from build123d import *

# Parameters (mm, degrees)
SKETCH2_R           = 12.954
BOSS_EXTRUDE1_DEPTH = 3.175
SKETCH3_R           = 5.969
BOSS_EXTRUDE2_DEPTH = 8.001
SKETCH4_R           = 2.794
SKETCH4_R_2         = 2.159
SKETCH4_R_3         = 1.397
BOSS_EXTRUDE3_DEPTH = 4.318


with BuildPart() as part:
    # Sketch2 → Boss-Extrude1 (new body)
    with BuildSketch(Plane(origin=(0, 0, 0), x_dir=(1, 0, 0), z_dir=(0, 1, 0))):
        with Locations(Location((0, 0, 0), (0, 0, 270))):
            Circle(SKETCH2_R)
    extrude(amount=BOSS_EXTRUDE1_DEPTH)

    # Sketch3 → Boss-Extrude2 (add)
    with BuildSketch(Plane(origin=(0, 3.175, 0), x_dir=(1, 0, 0), z_dir=(0, 1, 0))):
        with Locations(Location((0, 0, 0), (0, 0, 270))):
            Circle(SKETCH3_R)
    extrude(amount=BOSS_EXTRUDE2_DEPTH)

    # Sketch4 → Boss-Extrude3 (add)
    with BuildSketch(Plane(origin=(0, 11.176, 0), x_dir=(1, 0, 0), z_dir=(0, 1, 0))):
        with Locations(Location((0, 0, 0), (0, 0, 270))):
            Circle(SKETCH4_R)
        with Locations(Location((0, 0, 0), (0, 0, 270))):
            Circle(SKETCH4_R_2, mode=Mode.SUBTRACT)
        with Locations(Location((0, 0, 0), (0, 0, 270))):
            Circle(SKETCH4_R_3)
    extrude(amount=BOSS_EXTRUDE3_DEPTH)


solid = part.part
Design review of the part built by this model. Coordinates are the model's own, in mm. A direction names the side the tool comes from. Give positions to 0.01 mm unless a question says otherwise; leave off trailing zeros. Write each loop counter-clockwise with the first axis right and the second up, starting at its lowest first coordinate (ties: lowest second). Pieces come first, ordered by that corner, then holes. Notation, with made-up numbers: M 79,-14.75 L 87,-14.75 A26 cw 87,4.25 Z; hole C 55.5,51 d10. An arc over 180 degrees is marked long. Answer as a JSON object with one key per item and string values. Group by question number.
1) We need section D-D (y = 9.75). Give the boundary of the cut face in (x, z).
2) Tool access review of faces 1 (the face through (0, 0, 0)), 2 (the face through (-2.728, 13.305, -0.606)): name each direction out of +Z, -Z, +X, -X, +Y, -Y from which nothing blocks a thin tool from reaching the whole face with its end or side.
3) We need section C-C (x = 0). Give the boundary of the cut face in (y, z) (3 decimals), and give its area (3 significant figures).
4) For line 1 along X through (y, z) = (12.8, 0); line 2 along Z through (x, y) = (-0.5, 11.25); line 3 along Y through (x, z) = (-9.75, 5) (3 decimals), list the stretches that pass through material, from the lowest coordinate up.
5) We need section B-B (z = 0). Give the boundary of the cut face in (x, y) (3 decimals), and give its area (3 significant figures).
6) Clearance check with flat-ended pins moving along their axes: pin 1 Ø6 at (x, z) = (6.5, -8) entering from +Y (3 decimals); pin 2 Ø13 at (x, z) = (2, 5.5) entering from +Y; pin 3 Ø4 at (y, z) = (7, 1) entering from -X; pin 4 Ø6 at (x, y) = (4, 4) entering from -Z. State where each tip first meets the part, or that it passes through.
7) We need section A-A (y = 13). Give the boundary of the cut face in (x, z).
8) Mouldability with a two-part tool opening along X and no side actions: class faces 3 (the face through (1.793, 7.119, 5.693)), 4 (the face through (-1.364, 13.305, -0.303)), 5 (the face through (-1, 11.176, 3)) as released by +X, released by -X, zero draft, split by the parting line, or undercut.
Answer key:
{
 "1": {"outline": "C 0,0 d11.94"},
 "2": {"face 1": "+Z, -Z, +X, -X, -Y", "face 2": "+Y"},
 "3": {"outline": "M 0,-12.954 L 3.175,-12.954 L 3.175,-5.969 L 11.176,-5.969 L 11.176,-2.794 L 15.494,-2.794 L 15.494,-2.159 L 11.176,-2.159 L 11.176,-1.397 L 15.494,-1.397 L 15.494,1.397 L 11.176,1.397 L 11.176,2.159 L 15.494,2.159 L 15.494,2.794 L 11.176,2.794 L 11.176,5.969 L 3.175,5.969 L 3.175,12.954 L 0,12.954 Z", "area": "195 mm²"},
 "4": {"line 1": "x = -2.79 to -2.16, -1.4 to 1.4, 2.16 to 2.79", "line 2": "z = -2.75 to -2.1, -1.3 to 1.3, 2.1 to 2.75", "line 3": "y = 0 to 3.175"},
 "5": {"outline": "M -12.954,0 L 12.954,0 L 12.954,3.175 L 5.969,3.175 L 5.969,11.176 L 2.794,11.176 L 2.794,15.494 L 2.159,15.494 L 2.159,11.176 L 1.397,11.176 L 1.397,15.494 L -1.397,15.494 L -1.397,11.176 L -2.159,11.176 L -2.159,15.494 L -2.794,15.494 L -2.794,11.176 L -5.969,11.176 L -5.969,3.175 L -12.954,3.175 Z", "area": "195 mm²"},
 "6": {"pin 1": "stops at y = 3.175", "pin 2": "stops at y = 15.49", "pin 3": "stops at x = -5.97", "pin 4": "stops at z = -12.91"},
 "7": {"outline": "C 0,0 d5.59; C 0,0 d2.79; hole C 0,0 d4.32"},
 "8": {"face 3": "split by the parting line", "face 4": "undercut", "face 5": "zero draft"}
}
